from build123d import *

# Parameters (mm, degrees)
F0_W     = 90
F0_H     = 104
F0_R     = 2.1
F1_DEPTH = 5


with BuildPart() as f1:
    # F0 (on Front) → F1 (new body)
    with BuildSketch(Plane.XZ):
        Rectangle(F0_W, F0_H)
        with Locations((-32, -48)):
            Circle(F0_R, mode=Mode.SUBTRACT)
        with Locations((-24, -48)):
            Circle(F0_R, mode=Mode.SUBTRACT)
        with Locations((-32, -40)):
            Circle(F0_R, mode=Mode.SUBTRACT)
        with Locations((-40, -32)):
            Circle(F0_R, mode=Mode.SUBTRACT)
        with Locations((-32, -32)):
            Circle(F0_R, mode=Mode.SUBTRACT)
        with Locations((-16, -48)):
            Circle(F0_R, mode=Mode.SUBTRACT)
        with Locations((-8, -48)):
            Circle(F0_R, mode=Mode.SUBTRACT)
        with Locations((-40, -24)):
            Circle(F0_R, mode=Mode.SUBTRACT)
        with Locations((-40, -16)):
            Circle(F0_R, mode=Mode.SUBTRACT)
        with Locations((-40, -8)):
            Circle(F0_R, mode=Mode.SUBTRACT)
        with Locations((-8, -24)):
            Circle(F0_R, mode=Mode.SUBTRACT)
        with Locations((0, -48)):
            Circle(F0_R, mode=Mode.SUBTRACT)
        with Locations((8, -48)):
            Circle(F0_R, mode=Mode.SUBTRACT)
        with Locations((16, -48)):
            Circle(F0_R, mode=Mode.SUBTRACT)
        with Locations((24, -48)):
            Circle(F0_R, mode=Mode.SUBTRACT)
        with Locations((32, -48)):
            Circle(F0_R, mode=Mode.SUBTRACT)
        with Locations((32, -40)):
            Circle(F0_R, mode=Mode.SUBTRACT)
        with Locations((32, -32)):
            Circle(F0_R, mode=Mode.SUBTRACT)
        with Locations((40, -32)):
            Circle(F0_R, mode=Mode.SUBTRACT)
        with Locations((8, -24)):
            Circle(F0_R, mode=Mode.SUBTRACT)
        with Locations((40, -24)):
            Circle(F0_R, mode=Mode.SUBTRACT)
        with Locations((40, -16)):
            Circle(F0_R, mode=Mode.SUBTRACT)
        with Locations((40, -8)):
            Circle(F0_R, mode=Mode.SUBTRACT)
        with Locations((-40, 0)):
            Circle(F0_R, mode=Mode.SUBTRACT)
        with Locations((-40, 8)):
            Circle(F0_R, mode=Mode.SUBTRACT)
        with Locations((-40, 16)):
            Circle(F0_R, mode=Mode.SUBTRACT)
        with Locations((-40, 24)):
            Circle(F0_R, mode=Mode.SUBTRACT)
        with Locations((-8, 24)):
            Circle(F0_R, mode=Mode.SUBTRACT)
        with Locations((-40, 32)):
            Circle(F0_R, mode=Mode.SUBTRACT)
        with Locations((-32, 32)):
            Circle(F0_R, mode=Mode.SUBTRACT)
        with Locations((-32, 40)):
            Circle(F0_R, mode=Mode.SUBTRACT)
        with Locations((-32, 48)):
            Circle(F0_R, mode=Mode.SUBTRACT)
        with Locations((-24, 48)):
            Circle(F0_R, mode=Mode.SUBTRACT)
        with Locations((-16, 48)):
            Circle(F0_R, mode=Mode.SUBTRACT)
        with Locations((-8, 48)):
            Circle(F0_R, mode=Mode.SUBTRACT)
        with Locations((8, 24)):
            Circle(F0_R, mode=Mode.SUBTRACT)
        with Locations((40, 0)):
            Circle(F0_R, mode=Mode.SUBTRACT)
        with Locations((40, 8)):
            Circle(F0_R, mode=Mode.SUBTRACT)
        with Locations((40, 16)):
            Circle(F0_R, mode=Mode.SUBTRACT)
        with Locations((40, 24)):
            Circle(F0_R, mode=Mode.SUBTRACT)
        with Locations((0, 48)):
            Circle(F0_R, mode=Mode.SUBTRACT)
        with Locations((8, 48)):
            Circle(F0_R, mode=Mode.SUBTRACT)
        with Locations((16, 48)):
            Circle(F0_R, mode=Mode.SUBTRACT)
        with Locations((32, 32)):
            Circle(F0_R, mode=Mode.SUBTRACT)
        with Locations((40, 32)):
            Circle(F0_R, mode=Mode.SUBTRACT)
        with Locations((32, 40)):
            Circle(F0_R, mode=Mode.SUBTRACT)
        with Locations((24, 48)):
            Circle(F0_R, mode=Mode.SUBTRACT)
        with Locations((32, 48)):
            Circle(F0_R, mode=Mode.SUBTRACT)
    extrude(amount=F1_DEPTH)


solid = f1.part
Source: CAD feature listing. Evaluate the final solid. Frame: model axes, mm. Round coordinates to 2 decimals unless told otherwise and drop trailing zeros. Loops run counter-clockwise (first coordinate to the right, second up) from the corner with the lowest first, then second, coordinate; pieces in that order, holes last. Notation, with made-up numbers: (75, 78) - (115, 78) arc R25 cw to (115, 111) - close; hole circle Ø2 at (79, 12.5). An arc over 180 degrees is marked (long way). Write item = value, one per line. Start each with the question number.
Item 1: Mould query, pull axis X, two halves, no side actions, for faces 1 (the face through (-1, -5, 1)), 2 (the face through (30.334, -2.465, 38.722)). Classes: released by +X, released by -X, zero draft, split by the parting line, or undercut.
Item 2: Section query A-A on x = -16. Output: boundary loops of the cut face in (y, z), plus the area to 3 significant figures.
Item 3: Section query B-B on z = 8. Output: boundary loops of the cut face in (x, y).
Item 4: Material intervals for line 1 (Z direction, x = 0, y = -2.75); line 2 (Z direction, x = 8, y = -3.35); line 3 (X direction, y = -0.9, z = 7.5), sorted ascending.
Item 5: Section query D-D on y = -0.9. Count the separate pieces of the cut face and the enclosed holes in it, plus the area to 4 significant figures.
Item 6: Section query C-C on z = 32. Output: boundary loops of the cut face in (x, y).
Results list:
q1.face_1 = zero draft
q1.face_2 = undercut
q2.outline = (-5, -52) - (0, -52) - (0, -50.1) - (-5, -50.1) - close; (-5, -45.9) - (0, -45.9) - (0, 45.9) - (-5, 45.9) - close; (-5, 50.1) - (0, 50.1) - (0, 52) - (-5, 52) - close
q2.area = 478 mm²
q3.outline = (-45, -5) - (-42.1, -5) - (-42.1, 0) - (-45, 0) - close; (-37.9, -5) - (37.9, -5) - (37.9, 0) - (-37.9, 0) - close; (42.1, -5) - (45, -5) - (45, 0) - (42.1, 0) - close
q4.line_1 = -52 to -50.1, -45.9 to 45.9, 50.1 to 52
q4.line_2 = -52 to -50.1, -45.9 to -26.1, -21.9 to 21.9, 26.1 to 45.9, 50.1 to 52
q4.line_3 = -45 to -42.04, -37.96 to 37.96, 42.04 to 45
q5.separate_pieces = 1
q5.enclosed_holes = 48
q5.area = 8,695 mm²
q6.outline = (-45, -5) - (-42.1, -5) - (-42.1, 0) - (-45, 0) - close; (-37.9, -5) - (-34.1, -5) - (-34.1, 0) - (-37.9, 0) - close; (-29.9, -5) - (29.9, -5) - (29.9, 0) - (-29.9, 0) - close; (34.1, -5) - (37.9, -5) - (37.9, 0) - (34.1, 0) - close; (42.1, -5) - (45, -5) - (45, 0) - (42.1, 0) - close
